The figure shows three views and two pictorial views of one solid part (mm, origin at its lowest corner). Answer the questions. Give positions to 0.01 mm unless a question says otherwise; leave off trailing zeros. Order: outer loops, then holes, each group sorted by start corner. A loop starts at its lowest first (then second) coordinate and runs counter-clockwise, first axis right, second up. Notation, with made-up numbers: (14, 64) - (19, 64) arc R19 ccw to (19, 77) - close; hole circle Ø9 at (-13, -34.5). An arc over 180 degrees is marked (long way). Answer as CSV lines item,"result". Start each with the question number.
1. Flat-ended cylindrical pins translate along their axes: pin 1 (1.5 mm diameter, centred on y = 1, z = 58, fed in from +X); pin 2 (1.5 mm diameter, centred on x = 5, y = 1, fed in from -Z); pin 3 (0.9 mm diameter, centred on x = 38, y = 1.5, fed in from +Z). Find the tip coordinate at first contact, or state that the pin passes through.
2. Section A-A on z = 35 is taken. Give the vertices of the cut face in (x, y).
3. Section B-B on x = 36.5 is taken. Give the vertices of the cut face in (y, z).
4. Section D-D on x = 62 is taken. Give the vertices of the cut face in (y, z).
5. Consider line 1 along X through (y, z) = (0.7, 19.5); line 2 along Z through (x, y) = (51, 1.65); line 3 along X through (y, z) = (0.45, 51). Determine where each line is inside the solid, lowest interval first. Write a range as [from, to].
6. Section C-C on y = 2.1 is taken. Count the separate pieces of the cut face and the enclosed holes in it, and give its area (3 significant figures).
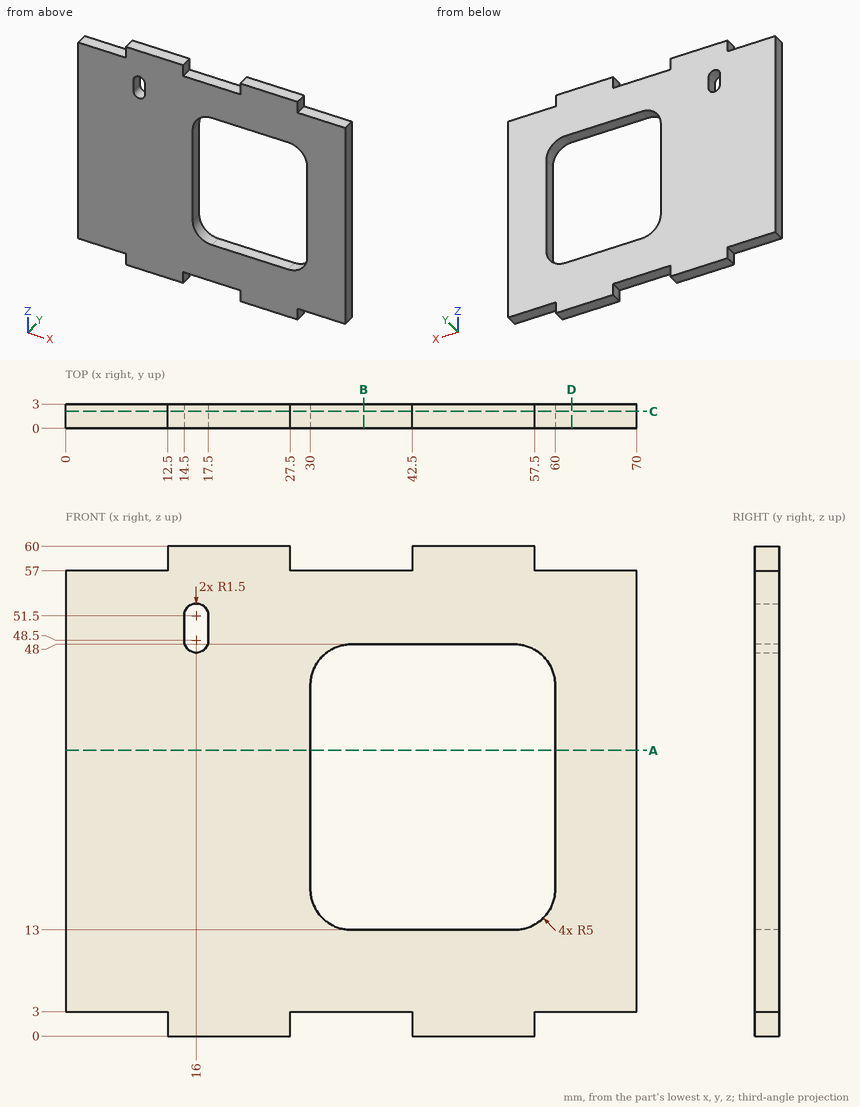
Checks:
1,pin 1,"stops at x = 57.5"
1,pin 2,"stops at z = 3"
1,pin 3,"stops at z = 57"
2,outline,"(0, 0) - (30, 0) - (30, 3) - (0, 3) - close; (60, 0) - (70, 0) - (70, 3) - (60, 3) - close"
3,outline,"(0, 3) - (3, 3) - (3, 13) - (0, 13) - close; (0, 48) - (3, 48) - (3, 57) - (0, 57) - close"
4,outline,"(0, 3) - (3, 3) - (3, 57) - (0, 57) - close"
5,line 1,"x = [0, 30], [60, 70]"
5,line 2,"z = [0, 13], [48, 60]"
5,line 3,"x = [0, 14.5], [17.5, 70]"
6,separate pieces,"1"
6,enclosed holes,"2"
6,area,"2,920 mm²"
